Autodesk Inventor part; units mm, degrees
ref_plane "YZ Plane" through (0, 0, 0) normal (1, 0, 0) x (0, 1, 0)
ref_plane "XZ Plane" through (0, 0, 0) normal (0, 1, 0) x (-1, 0, 0)
ref_plane "XY Plane" through (0, 0, 0) normal (0, 0, 1) x (1, 0, 0)
sketch "Sketch1" plane through (0, 0, 0) normal (1, 0, 0) x (0, 1, 0)
  circle A0 centre (0, 0) radius 25
  circle A1 centre (0, 0) radius 22
  line L0 (25, 0) -> (-25, 0)
  point P0 (-22, 0)
  point P1 (22, 0)
  dimension "d0" = 50
  dimension "d1" = 3
revolve "Revolution1" add sketch "Sketch1" angle 360 about axis through (0, 25, 0) along (0, -1, 0) picked at (23.7578, -1.9943) contours A0 L0 A1
split "Split1" plane through (0, 0, 0) removes the side toward (-1, 0, 0)
sketch "Sketch8" plane through (0, 0, 0) normal (-1, 0, 0) x (0, 0, 1)
  circle A0 centre (0, 0) radius 18
  dimension "d40" = 36
extrude "Extrusion7" cut sketch "Sketch8" against normal blind 39
chamfer "Chamfer1" distance 4 angle 45 1 edges at (17.3494, -0.0007, -18)
sketch "Sketch9" plane through (0, 0, 0) normal (-1, 0, 0) x (0, 0, 1)
  circle A0 centre (0, 0) radius 24
  circle A1 centre (0, 0) radius 23
  dimension "d46" = 48
  dimension "d47" = 1
extrude "Extrusion8" add sketch "Sketch9" along normal blind 3
sketch "Sketch10" plane through (0, 0, 0) normal (-1, 0, 0) x (0, 0, 1)
  line L0 (0, 0) -> (0, -25)
  circle A0 centre (0, 0) radius 25
  line L1 (7, -17.5) -> (-7, -17.5)
  line L2 (-7, -17.5) -> (-7, -32.5)
  line L3 (-7, -32.5) -> (7, -32.5)
  line L4 (7, -32.5) -> (7, -17.5)
  line L5 (7, -17.5) -> (-7, -32.5) construction
  line L6 (-7, -17.5) -> (7, -32.5) construction
  dimension "d50" = 14
  dimension "d51" = 15
extrude "Extrusion9" cut sketch "Sketch10" along normal mid plane 8 contours L1 L4 A0 L0 | L0 A0 L2 L1 | A0 L4 L3 L2
fillet "Fillet1" radius 2 1 edges at (14.2565, -0.0008, -20.5366)
properties part number "cover2"
The model under review builds one solid part; all positions refer to its coordinate system, in mm. A direction names the side the tool comes from. Coordinates: 2 decimals unless noted, no trailing zeros. Write each loop counter-clockwise with the first axis right and the second up, starting at its lowest first coordinate (ties: lowest second). Pieces come first, ordered by that corner, then holes. Notation, with made-up numbers: (10, 18) -> (53, 18) arc R31 ccw to (53, 50) -> close; hole circle Ø9 at (67, -11.5). An arc over 180 degrees is marked (long way). Answer in a Markdown table with one row per item.
1. For faces 1 (the cylindrical face through (12.994, 17.847, -2.343)), 2 (the flat face through (4, -23, 0)), 3 (the flat face through (0, 13.1, -20.3)), list the 3-axis set-ups (+Z, -Z, +X, -X, +Y, -Y) from which the entire face can be reached by the end or side of a thin tool; tool diameter is ignored.
Answers below:
| item | result |
|---|---|
| face 1 | +X, -X |
| face 2 | -X, -Y |
| face 3 | -X |
2. We need section B-B, the plane x = 1.5. State the section outline as (y, z) points.
Answers below:
| item | result |
|---|---|
| outline | (-23.95, -7) arc R24.95 ccw (long way) to (-23.95, 7) -> (-20.8, 7) arc R21.95 cw (long way) to (-20.8, -7) -> close |
3. Clearance check with flat-ended pins moving along their axes: pin 1 Ø3 at (x, y) = (0, -21.5) entering from -Z; pin 2 Ø12 at (y, z) = (6.5, -10.5) entering from +X; pin 3 Ø10 at (x, z) = (5, -6) entering from -Y. State where each tip first meets the part, or that it passes through.
Answers below:
| item | result |
|---|---|
| pin 1 | stops at z = -15 |
| pin 2 | stops at x = 13.47 |
| pin 3 | stops at y = -24.65 |
4. Wall thickness on probe 1 along Z at (x, y) = (-2, 0); probe 2 along Y at (x, z) = (-0.65, 0); probe 3 along Y at (x, z) = (7.5, -8): over which ranges is each line inside the solid? List them lowest first. Write a range as [from, to].
Answers below:
| item | result |
|---|---|
| probe 1 | z = [-24, -23], [23, 24] |
| probe 2 | y = [23, 24] |
| probe 3 | y = [-22.47, -19.07], [19.07, 22.47] |
5. Draft analysis for pull direction Y (two halves, no side actions). For faces 4 (the flat face through (1, -22, 7)), 5 (the flat face through (0, 19, -12)), 6 (the cylindrical face through (-1.48, 23.98, -0.96)), state which applies: +Y half, -Y half, draft (parallel to the pull), parting line (faces both ways), or undercut.
Answers below:
| item | result |
|---|---|
| face 4 | draft |
| face 5 | undercut |
| face 6 | parting line |
6. We need section A-A, the plane x = 8.5. State the section outline as (y, z) points, and give its area (3 significant figures).
Answers below:
| item | result |
|---|---|
| outline | circle Ø47.02 at (0, 0); hole circle Ø40.58 at (0, 0) |
| area | 443 mm^2 |
